Here's how the part is built. I have some questions about the finished solid (model axes, mm). Face numbers are marked on the shaded views. Coordinates: 2 decimals unless noted, no trailing zeros. Write each loop counter-clockwise with the first axis right and the second up, starting at its lowest first coordinate (ties: lowest second). Pieces come first, ordered by that corner, then holes.
Item 1: If we section it at A-A (x = -7.5): Please give me the cut outline in (y, z), then the cut area to 3 significant figures.
Item 2: If we section it at B-B (z = 12.7): Please give me the cut outline in (x, y), then the cut area to 3 significant figures.
Item 3: We'd pull the mould along Z, two halves only. Please class the marked faces 1, 2 and 3: +Z half, -Z half, draft (parallel to the pull), parting line (faces both ways), or undercut.
Item 4: I'm going to push flat-ended pins straight in: pin 1 Ø3.5 at (y, z) = (-5.848, 88.9) entering from +X; pin 2 Ø6 at (y, z) = (6.852, 88.9) entering from +X. Where does each tip first touch, or does it pass through?
Item 5: If I drill on line 1 (Y direction, x = -11.25, z = 12.7); line 2 (Y direction, x = -2.9, z = 88.9); line 3 (Z direction, x = -4.25, y = -4.5), over which ranges is the centre line in solid material (lowest first)?
Item 6: If we section it at C-C (y = -0.5): Please give me the cut outline in (x, z).
Item 7: If we section it at D-D (z = 69): Please give me the cut outline in (x, y).
Autodesk Inventor part; units mm, degrees
ref_plane "YZ Plane" through (0, 0, 0) normal (1, 0, 0) x (0, 1, 0)
ref_plane "XZ Plane" through (0, 0, 0) normal (0, 1, 0) x (-1, 0, 0)
ref_plane "XY Plane" through (0, 0, 0) normal (0, 0, 1) x (1, 0, 0)
sketch "Sketch1" plane through (0, 0, 0) normal (0, 0, 1) x (1, 0, 0)
  line L0 (-13.202, 13.202) -> (-0.502, 13.202)
  line L1 (-0.502, 13.202) -> (-0.502, -12.198)
  line L2 (-0.502, -12.198) -> (-13.202, -12.198)
  line L3 (-13.202, -12.198) -> (-13.202, 13.202)
  point P0 (0, 0)
  dimension "d0" = 12.7
  dimension "d1" = 25.4
extrude "Extrusion1" add sketch "Sketch1" along normal blind 101.6
sketch "Sketch6" plane through (-0.502, 13.202, 101.6) normal (1, 0, 0) x (0, 0, -1)
  line L0 (101.6, 0) -> (101.6, -25.4)
  line L1 (101.6, -25.4) -> (0, -25.4)
  line L2 (101.6, 0) -> (101.6, -25.4)
  line L3 (101.6, 0) -> (0, 0)
  line L4 (0, -25.4) -> (0, 0)
  line L5 (0, -25.4) -> (0, 0)
  point P0 (101.6, -13.202)
  point P1 (88.9, -6.35)
  point P2 (88.9, -19.05)
  point P3 (101.6, -19.05)
  point P4 (101.6, -6.35)
  point P5 (12.7, -6.35)
  point P6 (12.7, -19.05)
  point P7 (0, -19.05)
  point P8 (0, -6.35)
  dimension "d51" = 12.7
  dimension "d52" = 6.35
  dimension "d53" = 12.7
  dimension "d54" = 6.35
  dimension "d55" = 12.7
  dimension "d56" = 6.35
  dimension "d57" = 12.7
  dimension "d58" = 6.35
sketch "Sketch8" plane through (0, 0, 101.6) normal (0, 0, 1) x (1, 0, 0)
  line L0 (-13.202, 13.202) -> (-13.202, -12.198)
  line L1 (-13.202, -12.198) -> (-0.502, -12.198)
  point P0 (0, 0)
  point P1 (-5.582, 0.502)
  dimension "d82" = 7.62
  dimension "d84" = 12.7
hole "Hole4" at (-5.582, 0.502, 101.6) direction (0, 0, -1) diameter 6.477 end through all
hole "Hole5" at (-0.502, 6.852, 12.7) at (-0.502, -5.848, 12.7) at (-0.502, 6.852, 88.9) at (-0.502, -5.848, 88.9) direction (-1, 0, 0) diameter 4.318 end through all counterbore diameter 7.62 counterbore depth 4.318
properties part number "BottomOfElevatorFrameTop"
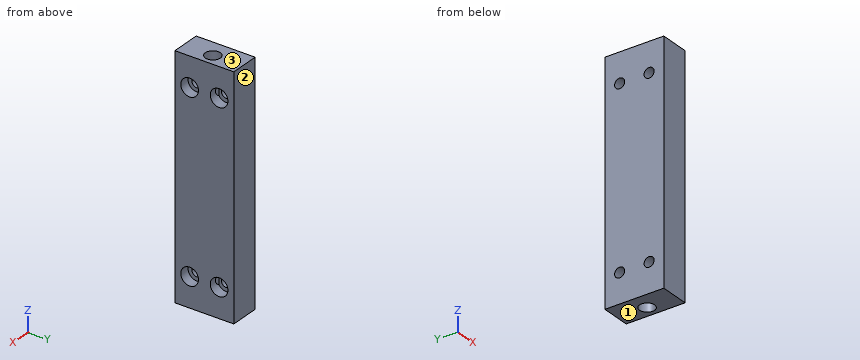
Answer list:
1. outline: (-12.2, 0) - (-2.11, 0) - (-2.11, 101.6) - (-12.2, 101.6) - close; (3.11, 0) - (13.2, 0) - (13.2, 101.6) - (3.11, 101.6) - close; hole circle Ø4.32 at (-5.85, 12.7); hole circle Ø4.32 at (-5.85, 88.9); hole circle Ø4.32 at (6.85, 12.7); hole circle Ø4.32 at (6.85, 88.9)
1. area: 1,990 mm2
2. outline: (-13.2, -12.2) - (-0.5, -12.2) - (-0.5, -9.66) - (-4.82, -9.66) - (-4.82, -8.01) - (-13.2, -8.01) - close; (-13.2, -3.69) - (-4.82, -3.69) - (-4.82, -2.65) arc R3.24 cw (long way) to (-4.82, 3.65) - (-4.82, 4.69) - (-13.2, 4.69) - close; (-13.2, 9.01) - (-4.82, 9.01) - (-4.82, 10.66) - (-0.5, 10.66) - (-0.5, 13.2) - (-13.2, 13.2) - close; (-3.57, -2.04) - (-0.5, -2.04) - (-0.5, 3.04) - (-3.57, 3.04) arc R3.24 cw to start
2. area: 152 mm2
3. face 1: -Z half
3. face 2: draft
3. face 3: +Z half
4. pin 1: passes through
4. pin 2: stops at x = -4.82
5. line 1: y = -12.2 to -8.01, -3.69 to 4.69, 9.01 to 13.2
5. line 2: y = -12.2 to -9.66, -2.04 to -1.31, 2.32 to 3.04, 10.66 to 13.2
5. line 3: z = 0 to 9.14, 16.26 to 85.34, 92.46 to 101.6
6. outline: (-13.2, 0) - (-8.66, 0) - (-8.66, 101.6) - (-13.2, 101.6) - close; (-2.5, 0) - (-0.5, 0) - (-0.5, 101.6) - (-2.5, 101.6) - close
7. outline: (-13.2, -12.2) - (-0.5, -12.2) - (-0.5, 13.2) - (-13.2, 13.2) - close; hole circle Ø6.48 at (-5.58, 0.5)
